Geometry check sheet. Reference: the model listing, model coordinates, mm. Face numbers are marked on the shaded views. A direction names the side the tool comes from. Coordinates: 2 decimals unless noted, no trailing zeros. Return JSON: item names as keys, results as strings. Group by question number.
Item 1: Draft check along Y on the marked faces 1 and 2. Enter one of: pulls with the +Y half, pulls with the -Y half, needs draft (parallel to the pull), parting line crosses it, or undercut.
Item 2: Section check A-A on z = 0. Give the number of separate pieces and of enclosed holes in the cut face, then the cut area to 3 significant figures.
Item 3: Scan lines: probe 1 along Z at (x, y) = (0, 21.9); probe 2 along Z at (x, y) = (0, 21); probe 3 along X at (y, z) = (57.5, 35.5). Record each from-to range of solid material in increasing order.
Item 4: Tool access check on the marked faces 3 and 4. Record the directions out of +Z, -Z, +X, -X, +Y, -Y that give a thin tool (end or side, any length) a straight path to the whole face; none if there is none.
Item 5: Gauge pin test, flat ends, axial feed: pin 1 (5 mm diameter, centred on y = -56, z = 0.5, fed in from +X); pin 2 (4 mm diameter, centred on x = -25.5, y = 44.5, fed in from +Z); pin 3 (3 mm diameter, centred on x = -66, y = -16.5, fed in from -Z); pin 4 (6 mm diameter, centred on x = -20, z = -25, fed in from -Y). Record the tip position at first contact, or that the pin passes through.
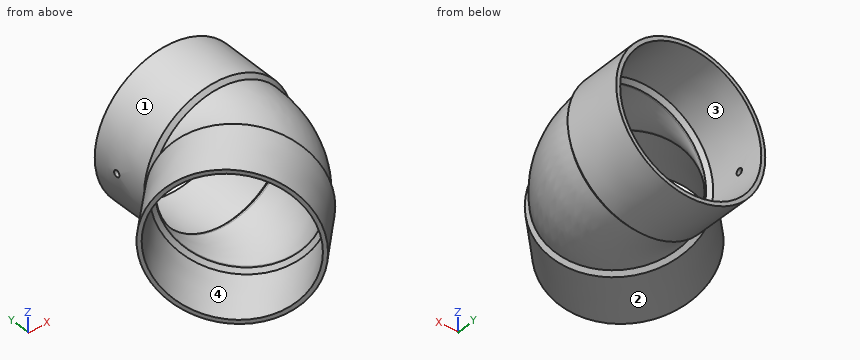
from build123d import *

# Parameters (mm, degrees)
SWEEP1_OUTLINE_R                 = 50.4825
SWEEP1_ANGLE                     = 45
F_10_0_1935_DIAMETER_HOLE1_D     = 4.9149
F_10_0_1935_DIAMETER_HOLE1_DEPTH = 76.2
F_10_0_1935_DIAMETER_HOLE1_TIP   = 1.476584928


# Read off the part's stored shape, not the designer's step: Sweep1
with BuildPart() as part:
    # Sketch1 → Revolve1 (revolve)
    with BuildSketch(Plane.XY):
        Polygon((-11.360023993, -87.422793339), (-9.204762524, -89.578054808), (22.903305281, -57.008000415), (22.873463107, -52.830095994), (20.718201637, -50.674834525), (19.81643184, -51.576604322), (19.846366028, -55.767390512), align=None)
    revolve(axis=Axis((-49.391408666, -49.391408666, 0), (0.707106781186549, 0.707106781186546, 0)))

    # Sketch2 → Revolve2 (revolve)
    with BuildSketch(Plane(origin=(0, 0, 0), x_dir=(-1, 0, 0), z_dir=(0, 0, -1)), mode=Mode.PRIVATE) as revolve2_sk:
        Polygon((-56.505826151, 24.1156612), (-53.5305, 21.182538256), (-50.4825, 21.182538256), (-50.4825, 22.457833333), (-53.467, 25.4), (-53.7845, 69.85), (-56.8325, 69.85), align=None)
    revolve(revolve2_sk.sketch.rotate(Axis((0, 69.85, 0), (0, -1, 0)), 180), axis=Axis((0, 69.85, 0), (0, -1, 0)))

    # Sweep1 outline → Sweep1 (revolve)
    with BuildSketch(Plane(origin=(-51.139171144, 21.182538256, 0), x_dir=(0.7071067811865458, -0.7071067811865492, 0), z_dir=(-0.7071067811865492, -0.7071067811865458, 0))):
        with BuildLine():
            add(Edge.make_bspline(
                [(0, -15.820859805), (3.386630847, -26.767767661), (10.25130148, -38.496554105), (21.767653092, -48.823978651), (37.04613395, -53.530499997), (58.423945129, -53.530500001), (65.508765494, -52.291102822), (71.965878454, -49.951324198), (77.591040871, -46.913712001), (89.454406147, -38.379551501), (96.226005165, -31.333524518), (101.848697911, -22.017553206), (107.472700853, 3.04e-07), (101.848697636, 22.017553663), (96.226004942, 31.333524749), (89.454406032, 38.379551584), (77.591040819, 46.913712039), (71.965878332, 49.951324264), (65.508765283, 52.291102899), (58.42394482, 53.530500055), (37.046133615, 53.530499893), (21.767652893, 48.823978477), (10.2513014, 38.496553967), (3.386630828, 26.767767599), (0, 15.820859805)],
                knots=[7.875906621, 7.875906621, 7.875906621, 7.875906621, 7.875906621, 7.875906621, 9.124748328, 9.124748328, 9.124748328, 9.124748328, 9.770281969, 9.770281969, 9.770281969, 9.770281969, 10.71746965, 10.71746965, 10.71746965, 11.664657316, 11.664657316, 11.664657316, 11.664657316, 12.310190963, 12.310190963, 12.310190963, 12.310190963, 13.559032663, 13.559032663, 13.559032663, 13.559032663, 13.559032663, 13.559032663], degree=5, weights=[1, 1, 0.991757982, 0.985412067, 1, 1, 0.999839694, 1.000222797, 1, 1, 0.999082466, 0.99680945, 1.00319055, 0.99680945, 0.999082467, 1, 1, 1.000222797, 0.999839694, 1, 1, 0.985412067, 0.991757982, 1, 1]))
            Line((0, 15.820859805), (0, -15.820859805))
        make_face()
        with Locations((51.139171144, 0)):
            Circle(SWEEP1_OUTLINE_R, mode=Mode.SUBTRACT)
    revolve(axis=Axis((-51.139171144, 21.182538256, 0), (0, 0, 1)), revolution_arc=SWEEP1_ANGLE)

    # #10 (0.1935) Diameter Hole1
    with Locations(Plane(origin=(-56.686954854, 49.473679541, 0), x_dir=(0.007142674934, -0.999974490772, 0), z_dir=(-0.999974490772, -0.007142674934, 0))):
        with Locations((0, 0)):
            Hole(F_10_0_1935_DIAMETER_HOLE1_D / 2, depth=F_10_0_1935_DIAMETER_HOLE1_DEPTH)
            with Locations((0, 0, -(F_10_0_1935_DIAMETER_HOLE1_DEPTH + F_10_0_1935_DIAMETER_HOLE1_TIP / 2))):  # 118° drill point
                Cone(0, F_10_0_1935_DIAMETER_HOLE1_D / 2, F_10_0_1935_DIAMETER_HOLE1_TIP, mode=Mode.SUBTRACT)


solid = part.part
Computed:
{
 "1": {"face 1": "undercut", "face 2": "parting line crosses it"},
 "2": {"separate pieces": "3", "enclosed holes": "0", "area": "837 mm²"},
 "3": {"probe 1": "z = -54.26 to -50.48, 50.48 to 54.26", "probe 2": "z = -53.53 to -50.48, 50.48 to 53.53", "probe 3": "x = -44.27 to -40.29, 40.29 to 44.27"},
 "4": {"face 3": "+Y", "face 4": "none"},
 "5": {"pin 1": "stops at x = 22.9", "pin 2": "stops at z = 51.55", "pin 3": "stops at z = -45.81", "pin 4": "passes through"}
}
